Here's how the part is built. I have some questions about the finished solid (model axes, mm). A direction names the side the tool comes from. Give positions to 0.01 mm unless a question says otherwise; leave off trailing zeros. Write each loop counter-clockwise with the first axis right and the second up, starting at its lowest first coordinate (ties: lowest second). Pieces come first, ordered by that corner, then holes. Notation, with made-up numbers: M 64,48 L 117,48 A8 cw 117,63 Z; hole C -39,24.5 d11. An arc over 180 degrees is marked long. Use one line per item in the form item = value. Start each with the question number.
Autodesk Inventor part; units mm, degrees
ref_plane "Work Plane1" through (164.5, 127, 270) normal (1, 0, 0) x (0, 0, 1)
ref_plane "XZ Plane" through (0, 0, 0) normal (0, 1, 0) x (-1, 0, 0)
ref_plane "XY Plane" through (0, 0, 0) normal (0, 0, 1) x (1, 0, 0)
sketch "Sketch1" plane through (0, 0, 0) normal (0, 0, 1) x (1, 0, 0)
  line L0 (0, 0) -> (100, 0)
  line L1 (100, 0) -> (100, 25)
  line L2 (100, 25) -> (0, 25)
  line L3 (0, 25) -> (0, 0)
  line L4 (0, 25) -> (115.2078, 140.2078)
  line L5 (100, 0) -> (177.7078, 77.7078)
  line L6 (151.2922, 176.2922) -> (200.5844, 163.0844)
  line L7 (200.5844, 163.0844) -> (213.7922, 113.7922)
  line L8 (213.7922, 113.7922) -> (177.7078, 77.7078)
  line L9 (177.7078, 77.7078) -> (128.4156, 90.9156)
  line L10 (128.4156, 90.9156) -> (115.2078, 140.2078)
  line L11 (115.2078, 140.2078) -> (151.2922, 176.2922)
  circle A0 centre (164.5, 127) radius 4
  dimension "d0" = 100
  dimension "d1" = 25
  dimension "d6" = 8
  dimension "d8" = 45
  dimension "d15" = 127
extrude "Extrusion1" add sketch "Sketch1" along normal blind 20
sketch "Sketch2" plane through (0, 0, 20) normal (0, 0, 1) x (1, 0, 0)
  line L0 (0, 25) -> (0, 0)
  line L1 (0, 0) -> (100, 0)
  line L2 (0, 25) -> (100, 25)
  line L3 (100, 25) -> (100, 0)
  line L4 (100, 0) -> (0, 0)
  line L5 (0, 0) -> (0, 25)
  line L6 (100, 25) -> (125, 25)
  line L7 (100, 0) -> (213.7922, 113.7922)
  line L8 (100, 0) -> (125, 25)
extrude "Extrusion2" add sketch "Sketch2" along normal blind 250
sketch "Sketch4" plane through (0, 0, 270) normal (0, 0, 1) x (1, 0, 0)
  line L0 (0, 25) -> (125, 25)
  line L1 (125, 25) -> (213.7922, 113.7922)
  line L2 (213.7922, 113.7922) -> (200.5844, 163.0844)
  line L3 (200.5844, 163.0844) -> (151.2922, 176.2922)
  line L4 (151.2922, 176.2922) -> (0, 25)
  circle A0 centre (164.5, 127) radius 4
  line L5 (100, 0) -> (125, 25)
  line L6 (125, 25) -> (0, 25)
  line L7 (0, 25) -> (0, 0)
  line L8 (0, 0) -> (100, 0)
extrude "Extrusion3" add sketch "Sketch4" along normal blind 20
sketch "Sketch5" plane through (0, 0, 0) normal (0, -1, 0) x (1, 0, 0)
  line L0 (0, 0) -> (100, 0)
  line L1 (100, 0) -> (100, 290)
  line L2 (0, 290) -> (100, 290)
  line L3 (0, 0) -> (0, 290)
  line L4 (0, 0) -> (-125.5737, 72.5)
  line L5 (-125.5737, 72.5) -> (-125.5737, 217.5)
  line L6 (-125.5737, 217.5) -> (0, 290)
  line L7 (0, 290) -> (125.5737, 217.5)
  line L8 (125.5737, 217.5) -> (125.5737, 72.5)
  line L9 (125.5737, 72.5) -> (0, 0)
  point P0 (0, 145)
extrude "Extrusion4" add sketch "Sketch5" against normal blind 25 contours L4 L5 L6 L3
sketch "Sketch6" plane through (0, 25, 20) normal (0, 1, 0) x (1, 0, 0)
  line L0 (100, 20) -> (100, -270)
  circle A0 centre (-24.528, -125) radius 3
  circle A1 centre (-31.528, -125) radius 1.5
  circle A2 centre (-21.028, -131.0622) radius 1.5
  circle A3 centre (-21.028, -118.9378) radius 1.5
  point P0 (0, 20)
  point P1 (100, -125)
  dimension "d18" = 6
  dimension "d19" = 124.528
  dimension "d20" = 3
  dimension "d21" = 7
  dimension "d24" = 360
extrude "Extrusion5" cut sketch "Sketch6" against normal through all
sketch "Sketch7" plane through (100, 0, 0) normal (0, -1, 0) x (1, 0, 0)
  circle A0 centre (-124.528, 145) radius 3
  circle A1 centre (-124.528, 145) radius 12
  point P0 (-100, 0)
  dimension "d28" = 24
extrude "Extrusion6" cut sketch "Sketch7" against normal blind 5
sketch "Sketch8" plane through (0, 0, 270) normal (0, 0, -1) x (-1, 0, 0)
  circle A0 centre (-164.5, 127) radius 4
  circle A1 centre (-164.5, 127) radius 12.5
  point P0 (0, 0)
  dimension "d31" = 25
extrude "Extrusion7" cut sketch "Sketch8" against normal blind 7
sketch "Sketch10" plane through (164.5, 127, 277) normal (0, 0, -1) x (-1, 0, 0)
  circle A0 centre (7, 0) radius 2
  circle A1 centre (0, 0) radius 4
  circle A2 centre (-3.5, 6.0622) radius 2
  circle A3 centre (-3.5, -6.0622) radius 2
  point P0 (164.5, -127)
  dimension "d34" = 4
  dimension "d37" = 360
  dimension "d39" = 7
extrude "Extrusion8" cut sketch "Sketch10" against normal through all
sketch "Sketch11" plane through (0, 0, 290) normal (0, 0, 1) x (1, 0, 0)
  circle A0 centre (168, 133.0622) radius 2
  circle A1 centre (164.5, 127) radius 4
  circle A2 centre (168, 133.0622) radius 4
  circle A3 centre (157.5, 127) radius 4
  circle A4 centre (168, 120.9378) radius 4
  point P0 (0, 0)
  dimension "d42" = 8
  dimension "d45" = 360
extrude "Extrusion9" cut sketch "Sketch11" against normal blind 3 contours A0 | A1 A4 A3 A2 | A2 A1 | A1 A2 | A4 A1 | A1 A4 | A3 A1 | A1 A3
ref_plane "Work Plane1" through (164.5, 127, 270) normal (1, 0, 0) x (0, 0, 1)
sketch "Sketch12" plane through (164.5, 127, 270) normal (1, 0, 0) x (0, 0, 1)
  line L0 (17, -1.9365) -> (17, 1.9365)
  line L1 (17, 1.9365) -> (20, 1.9365)
  line L2 (20, 3.9993) -> (20, 1.9365)
  line L3 (20, 3.9993) -> (17, 3.9993)
  line L4 (17, 3.9993) -> (17, 2.0628)
  line L5 (17, 2.0628) -> (20, 2.0628)
  line L6 (20, -2.0628) -> (20, 2.0628)
  line L7 (20, -2.0628) -> (17, -2.0628)
  line L8 (17, -2.0628) -> (17, -3.9993)
  line L9 (17, -3.9993) -> (20, -3.9993)
  line L10 (20, -1.9365) -> (20, -3.9993)
  line L11 (20, -1.9365) -> (17, -1.9365)
  line L12 (7, 4) -> (7, -4)
  line L13 (7, -12.5) -> (7, 12.5)
  line L14 (0, -12.5) -> (0, 12.5)
  circle A0 centre (3.5, 0) radius 2
  line L15 (0, -12.5) -> (7, -12.5)
  point P0 (-270, 127)
  point P1 (7, 0)
  point P2 (3.5, -12.5)
  dimension "d50" = 4
extrude "Extrusion10" cut sketch "Sketch12" along normal through all contours A0
sketch "Sketch13" plane through (0, 0, 20) normal (0, 0, 1) x (1, 0, 0)
  line L0 (100, 0) -> (213.7922, 113.7922)
  line L1 (213.7922, 113.7922) -> (200.5844, 163.0844)
  line L2 (200.5844, 163.0844) -> (151.2922, 176.2922)
  line L3 (151.2922, 176.2922) -> (0, 25)
  line L4 (0, 25) -> (0, 0)
  line L5 (0, 0) -> (100, 0)
  arc A0 (161, 128.9365) -> (161, 125.0635) centre (157.5, 127) ccw
  arc A1 (164.5729, 130.9993) -> (161, 128.9365) centre (164.5, 127) ccw
  arc A2 (167.9271, 129.0628) -> (164.5729, 130.9993) centre (168, 133.0622) ccw
  arc A3 (167.9271, 124.9372) -> (167.9271, 129.0628) centre (164.5, 127) ccw
  arc A4 (164.5729, 123.0007) -> (167.9271, 124.9372) centre (168, 120.9378) ccw
  arc A5 (161, 125.0635) -> (164.5729, 123.0007) centre (164.5, 127) ccw
  line L6 (-125.5737, 25) -> (0, 25)
  line L7 (0, 0) -> (-125.5737, 0)
  line L8 (0, 25) -> (0, 0)
  line L9 (-125.5737, 25) -> (0, 25)
  line L10 (-125.5737, 0) -> (-125.5737, 25)
extrude "Extrusion11" cut sketch "Sketch13" along normal through all contours L5 L4 L3 L2 L1 L0 | L7 L10 L6 L4 | A1 A2 A3 A4 A5 A0
sketch "Sketch14" plane through (0, 0, 20) normal (0, 0, 1) x (1, 0, 0)
  line L0 (-34.641, 0) -> (0, 0)
  line L1 (151.2922, 176.2922) -> (0, 25)
  line L2 (0, 0) -> (0, 25)
  line L3 (-34.641, 0) -> (-34.641, 25)
  line L4 (0, 25) -> (-34.641, 25)
  line L5 (-34.641, 25) -> (-34.641, 0)
  line L6 (-34.641, 0) -> (0, 0)
extrude "Extrusion12" cut sketch "Sketch14" against normal through all
sketch "Sketch15" plane through (0, 0, 20) normal (0, 0, 1) x (1, 0, 0)
  line L0 (15, 12.5) -> (90, 12.5) construction
  line L1 (0, 0) -> (100, 0)
  circle A0 centre (15, 12.5) radius 2.5
  circle A1 centre (90, 12.5) radius 2.5
  dimension "d57" = 75
  dimension "d58" = 12.5
  dimension "d59" = 10
  dimension "d60" = 5
  dimension "d61" = 5
extrude "Extrusion13" cut sketch "Sketch15" against normal through all
sketch "Sketch16" plane through (0, 0, 20) normal (0, 0, 1) x (1, 0, 0)
  circle A0 centre (164.5, 127) radius 4
  circle A1 centre (164.5, 127) radius 11.5
  point P0 (0, 0)
  dimension "d64" = 23
extrude "Extrusion14" cut sketch "Sketch16" against normal through all
sketch "Sketch17" plane through (0, 0, 20) normal (0, 0, 1) x (1, 0, 0)
  circle A0 centre (164.5, 127) radius 11.5
  circle A1 centre (164.5, 127) radius 22.5
  point P0 (0, 0)
  dimension "d67" = 45
extrude "Extrusion15" cut sketch "Sketch17" against normal blind 10
sketch "Sketch18" plane through (0, 0, 20) normal (0, 0, 1) x (1, 0, 0)
  circle A0 centre (62.5, 40) radius 7.5
  line L0 (0, 25) -> (0, 0)
  line L1 (0, 25) -> (125, 25)
  line L2 (100, 0) -> (213.7922, 113.7922)
  point P0 (62.5, 25)
  dimension "d70" = 15
  dimension "d71" = 15
extrude "Extrusion16" cut sketch "Sketch18" against normal through all
sketch "Sketch19" plane through (0, 0, 0) normal (0, 0, -1) x (-1, 0, 0)
  line L0 (-156.7794, 135.523) -> (-57.4648, 45.5585)
  circle A0 centre (-62.5, 40) radius 7.5
  line L1 (-67.1947, 34.1511) -> (-171.6985, 118.0316)
  circle A1 centre (-164.5, 127) radius 11.5
  circle A2 centre (-62.5, 40) radius 7.5
  arc A3 (-156.7794, 135.523) -> (-171.6985, 118.0316) centre (-164.5, 127) ccw
  arc A4 (-67.1947, 34.1511) -> (-57.4648, 45.5585) centre (-62.5, 40) ccw
  point P0 (0, 0)
extrude "Extrusion17" cut sketch "Sketch19" against normal blind 4
sketch "Sketch20" plane through (0, 0, 0) normal (0, 0, -1) x (-1, 0, 0)
  arc A0 (-156.7794, 135.523) -> (-171.6985, 118.0316) centre (-164.5, 127) ccw
  line L0 (-156.7794, 135.523) -> (-57.4648, 45.5585)
  line L1 (-67.1947, 34.1511) -> (-171.6985, 118.0316)
  arc A1 (-67.1947, 34.1511) -> (-57.4648, 45.5585) centre (-62.5, 40) ccw
  line L2 (-47.3944, 56.6755) -> (-146.709, 146.64)
  arc A2 (-146.709, 146.64) -> (-181.0879, 106.3338) centre (-164.5, 127) ccw
  line L3 (-181.0879, 106.3338) -> (-76.584, 22.4532)
  arc A3 (-76.584, 22.4532) -> (-47.3944, 56.6755) centre (-62.5, 40) ccw
  point P0 (0, 0)
  dimension "d76" = 15
extrude "Extrusion18" cut sketch "Sketch20" against normal blind 5 contours L0 A1 L1 A0 | A3 L3 A2 L2
sketch "Sketch21" plane through (0, 0, 5) normal (0, 0, -1) x (-1, 0, 0)
  circle A0 centre (-62.5, 40) radius 7.5
  circle A1 centre (-164.5, 127) radius 11.5
  line L0 (-146.709, 146.64) -> (-47.3944, 56.6755)
  arc A2 (-146.709, 146.64) -> (-181.0879, 106.3338) centre (-164.5, 127) ccw
  line L1 (-76.584, 22.4532) -> (-181.0879, 106.3338)
  arc A3 (-76.584, 22.4532) -> (-47.3944, 56.6755) centre (-62.5, 40) ccw
  line L2 (-76.584, 22.4532) -> (-181.0879, 106.3338)
  line L3 (-128.8359, 64.3935) -> (-97.0517, 101.6578) construction
  line L4 (-146.709, 146.64) -> (-47.3944, 56.6755)
  circle A4 centre (-125.5912, 68.1977) radius 2.5
  circle A5 centre (-100.2965, 97.8536) radius 2.5
  point P0 (0, 0)
  dimension "d79" = 5
  dimension "d80" = 5
  dimension "d81" = 5
  dimension "d82" = 5
extrude "Extrusion19" cut sketch "Sketch21" against normal through all contours A4 | A5
sketch "Sketch22" plane through (0, 0, 5) normal (0, 0, -1) x (-1, 0, 0)
  arc A0 (-146.709, 146.64) -> (-181.0879, 106.3338) centre (-164.5, 127) ccw
  arc A1 (-76.584, 22.4532) -> (-47.3944, 56.6755) centre (-62.5, 40) ccw
  line L0 (-180.8089, 140.9105) -> (-47.6313, 27.3179)
  line L1 (-76.584, 22.4532) -> (-181.0879, 106.3338)
  line L2 (-181.0879, 106.3338) -> (-180.8089, 140.9105)
  line L3 (-146.709, 146.64) -> (-180.8089, 140.9105)
  line L4 (-76.584, 22.4532) -> (-47.6313, 27.3179)
  line L5 (-47.3944, 56.6755) -> (-47.6313, 27.3179)
  point P0 (0, 0)
  dimension "d85" = 100
  dimension "d86" = 100
extrude "Extrusion20" add sketch "Sketch22" along normal blind 5 contours L3 L2 A0 | L4 L5 A1
properties part number "HA02" material "ABS Plastic"
1) Will these pins go through, and if not, where does the flat tip stop? P1, Ø1, axis at x = 89, y = 46.5, coming from the -Z side; P2, Ø6, axis at y = 144, z = 5.5, coming from the +X side; P3, Ø3, axis at x = 38.5, z = 4, coming from the +Y side; P4, Ø8, axis at x = 125.59, y = 68.2, coming from the +Z side.
2) Suppose I cut it at D-D, the plane y = 127. List the corners of the cut face in (x, z) for me, and give its area (3 significant figures).
3) Suppose I cut it at C-C, the plane z = 14.5. List the corners of the cut face in (x, y) for me.
4) On a 3-axis mill with a long thin cutter (end or side, diameter ignored), from which of +Z, -Z, +X, -X, +Y, -Y can I reach the whole of each face in a straight line? I mean faces 5 (the face through (176.6, 145.97, 15.07)), 6 (the face through (129.567, 64.981, 2.465)), 7 (the face through (105, 70, 20)). Say none if no direction works.
5) Suppose I cut it at A-A, the plane y = 12.5. List the corners of the cut face in (x, z) for me.
6) Suppose I cut it at B-B, the plane x = 90. List the corners of the cut face in (y, z) for me, and give its area (3 significant figures).
7) Please list where these lines run through material, in increasing order: line 1 (Z direction, x = 107, y = 106); line 2 (Y direction, x = 30, z = 4); line 3 (X direction, y = 43, z = 16.75).
8) Thinking about a two-plate mould opening in Y: for faces 1 (the face through (0, 12, 10)), 2 (the face through (207.096, 138.783, 9.86)), 3 (the face through (62.31, 24.85, 2.54)), 4 (the face through (115, 85, 5)), which applies, released by +Y, released by -Y, zero draft, split by the parting line, or undercut?
Checks:
q1.P1 = 5
q1.P2 = 206.5
q1.P3 = 65
q1.P4 = 20
q2.outline = M 102,0 L 125.03,0 L 125.03,5 L 153,5 L 153,10 L 142,10 L 142,20 L 102,20 Z; M 176,5 L 180.92,5 L 180.92,0 L 210.25,0 L 210.25,20 L 187,20 L 187,10 L 176,10 Z
q2.area = 1,320 mm^2
q3.outline = M 0,0 L 100,0 L 213.79,113.79 L 200.58,163.08 L 151.29,176.29 L 0,25 Z; hole C 15,12.5 d5; hole C 62.5,40 d15; hole C 90,12.5 d5; hole C 100.3,97.85 d5; hole C 125.59,68.2 d5; hole C 164.5,127 d45
q4.face_5 = +Z
q4.face_6 = -Z
q4.face_7 = +Z, +X, -X, +Y, -Y
q5.outline = M 0,0 L 12.5,0 L 12.5,20 L 0,20 Z; M 17.5,0 L 87.5,0 L 87.5,20 L 17.5,20 Z; M 92.5,0 L 112.5,0 L 112.5,20 L 92.5,20 Z
q6.outline = M 0,0 L 10,0 L 10,20 L 0,20 Z; M 15,0 L 33.22,0 L 33.22,5 L 95.27,5 L 95.27,0 L 115,0 L 115,20 L 15,20 Z
q6.area = 1,890 mm^2
q7.line_1 = 5 to 20
q7.line_2 = 0 to 55
q7.line_3 = 18 to 55.63, 69.37 to 143
q8.face_1 = zero draft
q8.face_2 = released by +Y
q8.face_3 = undercut
q8.face_4 = undercut
